Part model, mm, in its own coordinate system. A direction names the side the tool comes from. Give positions to 0.01 mm unless a question says otherwise; leave off trailing zeros. Write each loop counter-clockwise with the first axis right and the second up, starting at its lowest first coordinate (ties: lowest second). Pieces come first, ordered by that corner, then holes. Notation, with made-up numbers: M 74,2.5 L 118,2.5 A7 ccw 118,11.5 Z; hole C 22.25,-8.5 d7. An arc over 180 degrees is marked long. Use CSV: the item, a comma, the result in double quotes. Start each with the question number.
Item 1: Which spindle directions (+Z, -Z, +X, -X, +Y, -Y) get a long thin tool onto all of the face, cutting with end or side? Do faces 4 (the flat face through (-46.615, -17.319, -9.904)), 5 (the flat face through (-73.215, -18.738, -9.034)), 6 (the flat face through (43, 14.55, -7)), 7 (the flat face through (23, -6.55, 3)). Say none if no direction does.
Item 2: Cut at C-C (y = -17.55). List the corners of the cut face in (x, z) (3 decimals), then the cut area to 3 significant figures.
Item 3: Cut at D-D (x = 1). List the corners of the cut face in (y, z), then the cut area to 3 significant figures.
Item 4: Pin check, flat tips, straight feed: pin 1 (12 mm diameter, centred on y = -30.5, z = -7.5, fed in from +X); pin 2 (3 mm diameter, centred on x = 22.75, y = -4.5, fed in from -Z); pin 3 (1.2 mm diameter, centred on x = -82, z = -16.5, fed in from -Y); pin 4 (2 mm diameter, centred on x = 35, z = 2, fed in from -Y). Stop position of each tip, or through.
Item 5: Mould opens along Y. For faces 1 (the flat face through (-73, -50.296, -13)), 2 (the cylindrical face through (-46.615, -18.598, -14.013)), 3 (the flat face through (-46.615, 18.319, -9.904)) say: released by +Y, released by -Y, zero draft, split by the parting line, or undercut.
Item 6: Drill centre lines: line 1 (X direction, y = -11, z = -7.5); line 2 (X direction, y = -16.5, z = -12.5); line 3 (Z direction, x = -76.15, y = 13.5). Where is each one in solid material? Low to high. Write a range as [from, to].
Item 7: Cut at A-A (y = 4). List the corners of the cut face in (x, z) (3 decimals).
Item 8: Cut at B-B (z = -11.25). List the corners of the cut face in (x, y).
from build123d import *

# Parameters (mm, degrees)
SKETCH_1_W          = 40
SKETCH_1_H          = 30
EXTRUDE_1_DEPTH     = 15
SKETCH_3_R          = 1.55
EXTRUDE_2_DEPTH     = 5
SKETCH_4_W          = 6
SKETCH_4_H          = 4.77
EXTRUDE_3_DEPTH     = 4
SKETCH_5_W          = 129.3
SKETCH_5_H          = 30
SKETCH_5_W_2        = 13.8866
SKETCH_5_H_2        = 16
SKETCH_5_W_3        = 2.8866
EXTRUDE_4_DEPTH     = 4
SKETCH_7_R          = 1.55
SKETCH_7_W          = 4
SKETCH_7_H          = 0.95
SKETCH_7_H_2        = 28.1
EXTRUDE_5_DEPTH     = 4
SKETCH_8_R          = 1
EXTRUDE_6_DEPTH     = 5
EXTRUDE_7_DEPTH     = 5
EXTRUDE_8_DEPTH     = 4
SKETCH_12_R         = 1.05
CUT_EXTRUDE_1_DEPTH = 9
CUT_EXTRUDE_START   = -9
SKETCH_13_R         = 1.05
CUT_EXTRUDE_2_DEPTH = 9
CHAMFER_1_SIZE      = 7
CUT_EXTRUDE_3_REACH = 101.889
SKETCH_14_R         = 1
SKETCH_15_R         = 0.95
EXTRUDE_9_DEPTH     = 1
FILLET_1_R          = 0.5
CUT_EXTRUDE_4_DEPTH = 2.3


with BuildPart() as part:
    # Sketch 1 → Extrude 1 (new body)
    with BuildSketch(Plane.XY):
        with Locations((-64.15, 0.5)):
            Rectangle(SKETCH_1_W, SKETCH_1_H)
    extrude(amount=-EXTRUDE_1_DEPTH)

    # Sketch 3 → Extrude 2 (add)
    with BuildSketch(Plane(origin=(-44.15, 0, 0), x_dir=(0, 0, -1), z_dir=(1, 0, 0))):
        with BuildLine():
            Line((7.084541854, 15.5), (15, 15.5))
            Line((15, 15.5), (15, 15.003385417))
            ThreePointArc((15, 15.003385417), (18.463655357, 19.83658452), (12.644770927, 21.060229073))
            Line((12.644770927, 21.060229073), (7.084541854, 15.5))
        make_face()
        with Locations((15.155, 18.55)):
            Circle(SKETCH_3_R, mode=Mode.SUBTRACT)
    extrude_2 = extrude(amount=-EXTRUDE_2_DEPTH)

    # Mirror 2: Extrude 2 across plane
    add(extrude_2.mirror(Plane.ZX.offset(0.5)))

    # Sketch 4 → Extrude 3 (add)
    with BuildSketch(Plane(origin=(0, 0, -15), x_dir=(-1, 0, 0), z_dir=(0, 0, -1))):
        with Locations((47.15, 13.115)):
            Rectangle(SKETCH_4_W, SKETCH_4_H)
        with Locations((81.15, 13.115)):
            Rectangle(SKETCH_4_W, SKETCH_4_H)
        with Locations((81.15, -12.115)):
            Rectangle(SKETCH_4_W, SKETCH_4_H)
        with Locations((47.15, -12.115)):
            Rectangle(SKETCH_4_W, SKETCH_4_H)
    extrude(amount=EXTRUDE_3_DEPTH)

    # Sketch 5 → Extrude 4 (add)
    with BuildSketch(Plane.XY):
        with Locations((-19.5, 0.5)):
            Rectangle(SKETCH_5_W, SKETCH_5_H)
        with Locations((34.2067, 0)):
            Rectangle(SKETCH_5_W_2, SKETCH_5_H_2, mode=Mode.SUBTRACT)
        with Locations((-28.7067, 0)):
            Rectangle(SKETCH_5_W_3, SKETCH_5_H_2, mode=Mode.SUBTRACT)
    extrude(amount=EXTRUDE_4_DEPTH)

    # Sketch 7 → Extrude 5 (add)
    # profile 1 of 4: a face of its own
    with BuildSketch(Plane(origin=(45.15, 0, 0), x_dir=(0, 0, -1), z_dir=(1, 0, 0))):
        Polygon((19.155, -21.55), (19.155, -13.55), (15.155, -13.55), (0, -13.55), (0, -14.5), (-4, -14.5), (-4, -21.55), align=None)
        with Locations((15.155, -17.55)):
            Circle(SKETCH_7_R, mode=Mode.SUBTRACT)
    # profile 2 of 4: a face of its own
    with BuildSketch(Plane(origin=(45.15, 0, 0), x_dir=(0, 0, -1), z_dir=(1, 0, 0))):
        with Locations((-2, -14.025)):
            Rectangle(SKETCH_7_W, SKETCH_7_H)
    # profile 3 of 4: a face of its own
    with BuildSketch(Plane(origin=(45.15, 0, 0), x_dir=(0, 0, -1), z_dir=(1, 0, 0))):
        with Locations((17.155, 0.5)):
            Rectangle(SKETCH_7_W, SKETCH_7_H_2)
    # profile 4 of 4: a face of its own
    with BuildSketch(Plane(origin=(45.15, 0, 0), x_dir=(0, 0, -1), z_dir=(1, 0, 0))):
        Polygon((19.155, 14.55), (19.155, 22.55), (-4, 22.55), (-4, 15.5), (0, 15.5), (0, 14.55), (15.155, 14.55), align=None)
        with Locations((15.155, 18.55)):
            Circle(SKETCH_7_R, mode=Mode.SUBTRACT)
    extrude(amount=-EXTRUDE_5_DEPTH)

    # Sketch 8 → Extrude 6 (add)
    with BuildSketch(Plane(origin=(-75.679663749, 0, 0), x_dir=(0, 0, -1), z_dir=(1, 0, 0))):
        Polygon((13.392359313, -23.095757056), (18.235, -23.095757056), (18.235, -19.453116369), (13.281883631, -14.5), (4.796602257, -14.5), align=None)
        with Locations((15.235, -20.695757056)):
            Circle(SKETCH_8_R, mode=Mode.SUBTRACT)
    extrude(amount=EXTRUDE_6_DEPTH)



with BuildPart() as body_2:
    # Sketch 9 → Extrude 7 (new body)
    with BuildSketch(Plane(origin=(-75.679663749, 0, 0), x_dir=(0, 0, -1), z_dir=(1, 0, 0))):
        Polygon((-4, -39.331824868), (-4, -32.260757056), (9.335, -45.595757056), (9.335, -50.295757056), (6.963932188, -50.295757056), align=None)
        with BuildLine():
            Line((9.335, -45.595757056), (9.335, -50.295757056))
            Line((9.335, -50.295757056), (14.585, -50.295757056))
            Line((14.585, -50.295757056), (14.585, -48.755691264))
            ThreePointArc((14.585, -48.755691264), (14.816669987, -47.08746195), (16.235, -47.995757056))
            ThreePointArc((16.235, -47.995757056), (16.143295106, -48.41408707), (15.885, -48.755691264))
            Line((15.885, -48.755691264), (15.885, -50.295757056))
            Line((15.885, -50.295757056), (18.235, -50.295757056))
            Line((18.235, -50.295757056), (18.235, -45.595757056))
            Line((18.235, -45.595757056), (9.335, -45.595757056))
        make_face()
        with BuildLine():
            Line((14.585, -48.755691264), (14.585, -50.295757056))
            Line((14.585, -50.295757056), (15.885, -50.295757056))
            Line((15.885, -50.295757056), (15.885, -48.755691264))
            ThreePointArc((15.885, -48.755691264), (15.235, -48.995757056), (14.585, -48.755691264))
        make_face()
    extrude(amount=EXTRUDE_7_DEPTH)


with BuildPart() as part_1:
    add(part.part)

    add(body_2.part)  # Extrude 8 merges body 2
    # Sketch 11 → Extrude 8 (add)
    with BuildSketch(Plane.XY.offset(4)):
        Polygon((-70.679663749, -39.331824868), (-70.679663749, -22.970336251), (-62.209327497, -14.5), (-84.15, -14.5), (-75.679663749, -22.970336251), (-75.679663749, -39.331824868), align=None)
    extrude(amount=-EXTRUDE_8_DEPTH)

    # Sketch 12 → Cut-Extrude 1 (cut)
    with BuildSketch(Plane(origin=(0, 15.5, 0), x_dir=(1, 0, 0), z_dir=(0, 1, 0))):
        with Locations(Location((-76.15, 7.7, 0), (0, 0, 180))):
            Circle(SKETCH_12_R)
        with Locations(Location((-64.15, 7.7, 0), (0, 0, 180))):
            Circle(SKETCH_12_R)
    extrude(amount=-CUT_EXTRUDE_1_DEPTH, mode=Mode.SUBTRACT)

    # Sketch 13 → Cut-Extrude 2 (cut)
    with BuildSketch(Plane.XZ.offset(14.5).offset(CUT_EXTRUDE_START)):
        with Locations(Location((-64.15, -7.7, 0), (0, 0, 180))):
            Circle(SKETCH_13_R)
        with Locations((-79.652663002, -7.7)):
            Circle(SKETCH_13_R)
    extrude(amount=CUT_EXTRUDE_2_DEPTH, mode=Mode.SUBTRACT)

    # Chamfer 1
    chamfer_1_edges = [part_1.edges().sort_by_distance(p)[0] for p in [
        (41.15, -14.5, 2),
        (41.15, 15.5, 2),
    ]]
    chamfer(chamfer_1_edges, length=CHAMFER_1_SIZE)

    # Sketch 14 → Cut-Extrude 3 (cut, up to next)
    with BuildSketch(Plane(origin=(0, 0, 0), x_dir=(-1, 0, 0), z_dir=(0, 0, -1)), mode=Mode.PRIVATE) as cut_extrude_3_sk1:
        with Locations((-22.75, -4.5)):
            Circle(SKETCH_14_R)
    cut_extrude_3_tool1 = extrude(cut_extrude_3_sk1.sketch, amount=-CUT_EXTRUDE_3_REACH, mode=Mode.PRIVATE) & part_1.part
    # Sketch 14 → Cut-Extrude 3 (cut, up to next)
    with BuildSketch(Plane(origin=(0, 0, 0), x_dir=(-1, 0, 0), z_dir=(0, 0, -1)), mode=Mode.PRIVATE) as cut_extrude_3_sk2:
        with Locations((13.65, -4.5)):
            Circle(SKETCH_14_R)
    cut_extrude_3_tool2 = extrude(cut_extrude_3_sk2.sketch, amount=-CUT_EXTRUDE_3_REACH, mode=Mode.PRIVATE) & part_1.part
    add(cut_extrude_3_tool1.solids().sort_by_distance((22.75, -4.5, 0))[0], mode=Mode.SUBTRACT)
    add(cut_extrude_3_tool2.solids().sort_by_distance((-13.65, -4.5, 0))[0], mode=Mode.SUBTRACT)

    # Sketch 15 → Extrude 9 (add)
    with BuildSketch(Plane(origin=(0, 0, 0), x_dir=(-1, 0, 0), z_dir=(0, 0, -1))):
        with Locations((18.27, -4.5)):
            Circle(SKETCH_15_R)
        with Locations((-18.1, -4.5)):
            Circle(SKETCH_15_R)
    extrude(amount=EXTRUDE_9_DEPTH)

    # Fillet 1
    fillet_1_edges = [part_1.edges().sort_by_distance(p)[0] for p in [
        (-17.32, -4.5, -1),
        (19.05, -4.5, -1),
    ]]
    fillet(fillet_1_edges, radius=FILLET_1_R)

    # Sketch 16 → Cut-Extrude 4 (cut)
    with BuildSketch(Plane.XY.offset(4)):
        Polygon((25.117136104, -4.5), (23.933568052, -2.45), (21.566431948, -2.45), (20.382863896, -4.5), (21.566431948, -6.55), (23.933568052, -6.55), align=None)
        Polygon((-11.282863896, -4.5), (-12.466431948, -2.45), (-14.833568052, -2.45), (-16.017136104, -4.5), (-14.833568052, -6.55), (-12.466431948, -6.55), align=None)
    extrude(amount=-CUT_EXTRUDE_4_DEPTH, mode=Mode.SUBTRACT)


solid = part_1.part
Worked answers:
1,face 4,"+Z, -Y"
1,face 5,"-X"
1,face 6,"+X"
1,face 7,"+Z"
2,outline,"M -81.1,0 L -65.259,0 L -65.259,4 L -81.1,4 Z; M -75.68,-16.332 L -70.68,-16.332 L -70.68,-7.847 L -75.68,-7.847 Z; M -49.15,-18.705 L -44.15,-18.705 L -44.15,-16.705 L -49.15,-16.705 Z; M -49.15,-13.605 L -44.15,-13.605 L -44.15,-10.135 L -49.15,-10.135 Z; M 37.2,0 L 41.15,0 L 41.15,-13.605 L 45.15,-13.605 L 45.15,4 L 37.2,4 Z; M 41.15,-19.155 L 45.15,-19.155 L 45.15,-16.705 L 41.15,-16.705 Z"
2,area,"229 mm^2"
3,outline,"M -14.5,0 L 15.5,0 L 15.5,4 L -14.5,4 Z"
3,area,"120 mm^2"
4,pin 1,"passes through"
4,pin 2,"stops at z = 0"
4,pin 3,"stops at y = -14.5"
4,pin 4,"stops at y = -16.35"
5,face 1,"released by -Y"
5,face 2,"undercut"
5,face 3,"released by +Y"
6,line 1,"x = [-84.15, -80.68], [-78.62, -65.18], [-63.12, -44.15]"
6,line 2,"x = [-75.68, -70.68], [-49.15, -44.15], [41.15, 45.15]"
6,line 3,"z = [-15, -8.75], [-6.65, 4]"
7,outline,"M -84.15,-15 L -44.15,-15 L -44.15,0 L -30.15,0 L -30.15,4 L -84.15,4 Z; M -27.263,0 L 27.263,0 L 27.263,4 L -27.263,4 Z; M 41.15,-19.155 L 45.15,-19.155 L 45.15,-15.155 L 41.15,-15.155 Z; M 41.15,0 L 45.15,0 L 45.15,4 L 41.15,4 Z"
8,outline,"M -84.15,-14.5 L -75.68,-14.5 L -75.68,-20.95 L -70.68,-20.95 L -70.68,-14.5 L -49.15,-14.5 L -49.15,-18.67 L -44.15,-18.67 L -44.15,19.67 L -49.15,19.67 L -49.15,15.5 L -84.15,15.5 Z; M -75.68,-50.3 L -70.68,-50.3 L -70.68,-45.6 L -75.68,-45.6 Z; M 41.15,-21.55 L 45.15,-21.55 L 45.15,-13.55 L 41.15,-13.55 Z; M 41.15,14.55 L 45.15,14.55 L 45.15,22.55 L 41.15,22.55 Z"
